Model file for the job. Use its own axes, mm. A direction names the side the tool comes from. Round coordinates to 2 decimals unless told otherwise and drop trailing zeros. Loops run counter-clockwise (first coordinate to the right, second up) from the corner with the lowest first, then second, coordinate; pieces in that order, holes last. Notation, with made-up numbers: M 80.5,-30 L 136.5,-30 A15 cw 136.5,-23 Z; hole C 88.5,41 d2. An arc over 180 degrees is marked long. Use a Markdown table: item, result. Add a question column.
Q1. Tool access for faces 1 (the face through (-52, 2, 7.5)), 2 (the face through (-9.66, 2, 0)), 3 (the face through (52, 2, -7.5)): list every direction of +Z, -Z, +X, -X, +Y, -Y with a clear straight run to the whole face (end or side of a thin tool).
Q2. Cut at D-D (z = 13.25). Give the cut face in (x, y).
Q3. Pin check, flat tips, straight feed: pin 1 (1.6 mm diameter, centred on y = 2, z = 9.5, fed in from +X); pin 2 (6.5 mm diameter, centred on x = -13.47, z = -5.085, fed in from -Y); pin 3 (1 mm diameter, centred on x = -52.5, y = 1.5, fed in from +Z); pin 4 (1.6 mm diameter, centred on y = 1, z = -10.5, fed in from -X). Stop position of each tip, or through.
Q4. Cut at B-B (x = 26). Give the cut face in (y, z).
Q5. Cut at A-A (x = -13.47). Give the cut face in (y, z) (3 decimals), plus the area to 3 significant figures.
Q6. Probe line 1 (Z direction, x = -13.47, y = 1.15) (3 decimals); line 2 (X direction, y = 0.8, z = 8.75); line 3 (Z direction, x = 20, y = 0.5). List the from-to ranges inside material, lowest first. Write a range as from..to.
Q7. Cut at C-C (y = 1). Give the cut face in (x, z) (3 decimals), plus the area to 3 significant figures.
Autodesk Inventor part; units mm, degrees
ref_plane "YZ Plane" through (0, 0, 0) normal (1, 0, 0) x (0, 1, 0)
ref_plane "XZ Plane" through (0, 0, 0) normal (0, 1, 0) x (-1, 0, 0)
ref_plane "XY Plane" through (0, 0, 0) normal (0, 0, 1) x (1, 0, 0)
sketch "Boceto2" plane through (0, 0, 0) normal (0, 1, 0) x (-1, 0, 0)
  circle A0 centre (0, 0) radius 5
  line L0 (9.66, 9.91) -> (-30.22, 9.91)
  line L1 (-30.22, 9.91) -> (-30.22, -9.91)
  line L2 (-30.22, -9.91) -> (9.66, -9.91)
  line L3 (9.66, -9.91) -> (9.66, 9.91)
  circle A1 centre (-33.79, 5.085) radius 2
  circle A2 centre (13.47, -5.085) radius 2
  circle A3 centre (13.47, 5.085) radius 2
  circle A4 centre (-33.79, -5.085) radius 2
  line L4 (-50, 15) -> (50, 15)
  line L5 (50, 15) -> (50, -15)
  line L6 (50, -15) -> (-50, -15)
  line L7 (-50, -15) -> (-50, 15)
  line L8 (-50, 15) -> (50, -15) construction
  line L9 (50, 15) -> (-50, -15) construction
  line L10 (53.18, 7.5) -> (50, 7.5)
  line L11 (50, 7.5) -> (50, -7.5)
  line L12 (50, -7.5) -> (53.18, -7.5)
  line L13 (53.18, -7.5) -> (53.18, 7.5)
  line L14 (-50, 7.5) -> (-53.18, 7.5)
  line L15 (-53.18, 7.5) -> (-53.18, -7.5)
  line L16 (-53.18, -7.5) -> (-50, -7.5)
  line L17 (-50, -7.5) -> (-50, 7.5)
  dimension "d2" = 10
  dimension "d3" = 9.91
  dimension "d4" = 19.82
  dimension "d5" = 9.66
  dimension "d6" = 39.88
  dimension "d7" = 4
  dimension "d8" = 4
  dimension "d9" = 4
  dimension "d10" = 5.085
  dimension "d11" = 10.17
  dimension "d12" = 13.47
  dimension "d13" = 13.47
  dimension "d14" = 4
  dimension "d15" = 33.79
  dimension "d16" = 33.79
  dimension "d17" = 5.085
  dimension "d18" = 10.17
  dimension "d19" = 100
  dimension "d20" = 30
  dimension "d21" = 3.18
  dimension "d22" = 15
  dimension "d23" = 7.5
  dimension "d24" = 15
  dimension "d25" = 3.18
  dimension "d26" = 7.5
extrude "Extrusión1" add sketch "Boceto2" along normal blind 3.18 contours L4 L5 L6 L7 | L7 L16 L15 L14 | L10 L13 L12 L5
properties part number "BASE_SOST.SERVO"
Checked values:
| question | item | result |
|---|---|---|
| 1 | face 1 | +Z, -X, +Y, -Y |
| 1 | face 2 | +Y, -Y |
| 1 | face 3 | -Z, +X, +Y, -Y |
| 2 | outline | M -50,0 L 50,0 L 50,3.18 L -50,3.18 Z |
| 3 | pin 1 | stops at x = 50 |
| 3 | pin 2 | stops at y = 0 |
| 3 | pin 3 | stops at z = 7.5 |
| 3 | pin 4 | stops at x = -50 |
| 4 | outline | M 0,-15 L 3.18,-15 L 3.18,-9.91 L 0,-9.91 Z; M 0,9.91 L 3.18,9.91 L 3.18,15 L 0,15 Z |
| 5 | outline | M 0,-15 L 3.18,-15 L 3.18,-7.085 L 0,-7.085 Z; M 0,-3.085 L 3.18,-3.085 L 3.18,3.085 L 0,3.085 Z; M 0,7.085 L 3.18,7.085 L 3.18,15 L 0,15 Z |
| 5 | area | 70.0 mm^2 |
| 6 | line 1 | z = -15..-7.085, -3.085..3.085, 7.085..15 |
| 6 | line 2 | x = -50..-9.66, 30.22..50 |
| 6 | line 3 | z = -15..-9.91, 9.91..15 |
| 7 | outline | M -53.18,-7.5 L -50,-7.5 L -50,-15 L 50,-15 L 50,-7.5 L 53.18,-7.5 L 53.18,7.5 L 50,7.5 L 50,15 L -50,15 L -50,7.5 L -53.18,7.5 Z; hole C -13.47,-5.085 d4; hole C -13.47,5.085 d4; hole M -9.66,-9.91 L 30.22,-9.91 L 30.22,9.91 L -9.66,9.91 Z; hole C 33.79,-5.085 d4; hole C 33.79,5.085 d4 |
| 7 | area | 2,250 mm^2 |
